The listing builds one solid part. Answer for the finished solid, in the listing's coordinates (mm). A direction names the side the tool comes from. Give positions to 0.01 mm unless a question says otherwise; leave off trailing zeros. Order: outer loops, then holes, each group sorted by start corner. A loop starts at its lowest first (then second) coordinate and runs counter-clockwise, first axis right, second up. Notation, with made-up numbers: (19.5, 34) - (23.5, 34) arc R19 ccw to (23.5, 39) - close; hole circle Ø7 at (66.25, 46). An arc over 180 degrees is marked (long way). Use CSV: the item, a comma, the result in double quotes.
```python
from build123d import *

# Parameters (mm, degrees)
F0_W     = 25.4
F0_H     = 25.4
F1_DEPTH = 22.225
F2_W     = 19.05
F2_H     = 19.05
F3_DEPTH = 15.875
F4_R     = 2.54


with BuildPart() as f1:
    # F0 (on Top) → F1 (new body)
    with BuildSketch(Plane.XY):
        with Locations((12.7, 12.7)):
            Rectangle(F0_W, F0_H)
    extrude(amount=F1_DEPTH)

    # F2 (on face) → F3 (cut)
    with BuildSketch(Plane(origin=(0, 0, 0), x_dir=(1, 0, 0), z_dir=(0, 0, -1))):
        with Locations((12.7, -12.7)):
            Rectangle(F2_W, F2_H)
    extrude(amount=-F3_DEPTH, mode=Mode.SUBTRACT)

    # F4
    f4_edges = [f1.edges().sort_by_distance(p)[0] for p in [
        (25.4, 0, 11.1125),
        (25.4, 25.4, 11.1125),
        (0, 25.4, 11.1125),
        (0, 0, 11.1125),
    ]]
    fillet(f4_edges, radius=F4_R)


solid = f1.part
```
Item 1: The mould has two halves that part along X. Classify faces 1 (the face through (13, 0, 11)), 2 (the face through (13, 13, 15.875)), 3 (the face through (0.724, 0.764, 11.268)): +X half, -X half, draft (parallel to the pull), parting line (faces both ways), or undercut.
Taken from the geometry:
face 1,"draft"
face 2,"undercut"
face 3,"-X half"
Item 2: This flat-tipped pin is pushed along its axis until it touches: pin 1 (10 mm diameter, centred on x = 15, y = 6, fed in from -Z). Where does it stop, or does it pass through?
Taken from the geometry:
pin 1,"z = 0"
Item 3: The part is cut by section A-A (y = 5). Give the vertices of the cut face in (x, z) (3 decimals).
Taken from the geometry:
outline,"(0, 0) - (3.175, 0) - (3.175, 15.875) - (22.225, 15.875) - (22.225, 0) - (25.4, 0) - (25.4, 22.225) - (0, 22.225) - close"
Item 4: Find the intervals of material crossed by line 1 along Y through (x, z) = (10.75, 7.5) (3 decimals); line 2 along Z through (x, y) = (7, 14.5) (3 decimals), in increasing order.
Taken from the geometry:
line 1,"0 to 3.175, 22.225 to 25.4"
line 2,"15.875 to 22.225"
Item 5: The part is cut by section B-B (z = 15). Give the vertices of the cut face in (x, y) (3 decimals).
Taken from the geometry:
outline,"(0, 2.54) arc R2.54 ccw to (2.54, 0) - (22.86, 0) arc R2.54 ccw to (25.4, 2.54) - (25.4, 22.86) arc R2.54 ccw to (22.86, 25.4) - (2.54, 25.4) arc R2.54 ccw to (0, 22.86) - close; hole (3.175, 3.175) - (22.225, 3.175) - (22.225, 22.225) - (3.175, 22.225) - close"
Item 6: Which of the six approach directions +Z, -Z, +X, -X, +Y, -Y give full straight-line access (tool end or side, diameter ignored) to faces 4 (the face through (24.636, 24.676, 11.268)), 5 (the face through (13, 22.225, 8))?
Taken from the geometry:
face 4,"+Z, -Z, +X, +Y"
face 5,"-Z"
